from build123d import *

# Parameters (mm, degrees)
F2_R      = 51.5
F2_R_2    = 49
F5_DEPTH  = 10
F7_R      = 2.5
F8_DEPTH  = 5
F9_W      = 160.924614
F9_H      = 163.103462
F9_W_2    = 140
F9_H_2    = 140
F10_DEPTH = 10


with BuildPart() as f4:
    # F3 (on Front) → F4 (revolve)
    with BuildSketch(Plane.XZ):
        with BuildLine():
            ThreePointArc((63.105709, 14.230078), (67.468124, 7.701262), (69, 0))
            Line((69, 0), (72.5, 0))
            ThreePointArc((72.5, 0), (71.091539, 7.08081), (67.080583, 13.083631))
            Line((67.080583, 13.083631), (59.515611, 20.648602))
            ThreePointArc((59.515611, 20.648602), (53.58319, 29.527099), (51.5, 40))
            Line((51.5, 40), (45, 40))
            ThreePointArc((45, 40), (46.408461, 32.91919), (50.419417, 26.916369))
            Line((50.419417, 26.916369), (63.105709, 14.230078))
        make_face()
    revolve(axis=Axis((0, 0, 20), (0, 0, 1)))

    # F2 (on offset) → F5 (join)
    with BuildSketch(Plane.XY.offset(40)):
        Circle(F2_R)
        Circle(F2_R_2, mode=Mode.SUBTRACT)
    extrude(amount=F5_DEPTH)

    # F7 (on offset) → F8 (join)
    with BuildSketch(Plane.XY.offset(5)):
        with BuildLine():
            Line((-70, 65), (-70, 16.028423))
            ThreePointArc((-70, 16.028423), (-50.778491, 50.778491), (-16.028423, 70))
            Line((-16.028423, 70), (-65, 70))
            ThreePointArc((-65, 70), (-68.535534, 68.535534), (-70, 65))
        make_face()
        with Locations((-62.25, 62.25)):
            Circle(F7_R, mode=Mode.SUBTRACT)
        with BuildLine():
            ThreePointArc((-16.028423, -70), (-50.778491, -50.778491), (-70, -16.028423))
            Line((-70, -16.028423), (-70, -65))
            ThreePointArc((-70, -65), (-68.535534, -68.535534), (-65, -70))
            Line((-65, -70), (-16.028423, -70))
        make_face()
        with Locations((-62.25, -62.25)):
            Circle(F7_R, mode=Mode.SUBTRACT)
        with BuildLine():
            ThreePointArc((70, -16.028423), (50.778491, -50.778491), (16.028423, -70))
            Line((16.028423, -70), (65, -70))
            ThreePointArc((65, -70), (68.535534, -68.535534), (70, -65))
            Line((70, -65), (70, -16.028423))
        make_face()
        with Locations((62.25, -62.25)):
            Circle(F7_R, mode=Mode.SUBTRACT)
        with BuildLine():
            Line((65, 70), (16.028423, 70))
            ThreePointArc((16.028423, 70), (50.778491, 50.778491), (70, 16.028423))
            Line((70, 16.028423), (70, 65))
            ThreePointArc((70, 65), (68.535534, 68.535534), (65, 70))
        make_face()
        with Locations((62.25, 62.25)):
            Circle(F7_R, mode=Mode.SUBTRACT)
    extrude(amount=-F8_DEPTH)

    # F9 (on Top) → F10 (cut)
    with BuildSketch(Plane.XY):
        Rectangle(F9_W, F9_H)
        Rectangle(F9_W_2, F9_H_2, mode=Mode.SUBTRACT)
    extrude(amount=F10_DEPTH, mode=Mode.SUBTRACT)


solid = f4.part
Verification items for the finished model (mm, model axes). A direction names the side the tool comes from. Coordinates: 2 decimals unless noted, no trailing zeros. Order: outer loops, then holes, each group sorted by start corner. A loop starts at its lowest first (then second) coordinate and runs counter-clockwise, first axis right, second up.
Item 1: Material ranges on L1, parallel to Y at x = 62.25, z = 2.95; L2, parallel to Y at x = 62.25, z = 2.8; L3, parallel to Z at x = -59, y = 59, recorded low to high.
Filled in:
L1: y = -70 to -64.75, -59.75 to -29.26, 29.26 to 59.75, 64.75 to 70
L2: y = -70 to -64.75, -59.75 to -29.31, 29.31 to 59.75, 64.75 to 70
L3: z = 0 to 5
Item 2: Depth check by flat-ended pin: pin 1 (4 mm diameter, centred on x = 15.5, z = 9.5, fed in from +Y); pin 2 (2 mm diameter, centred on x = -35, y = -43.5, fed in from -Z); pin 3 (8 mm diameter, centred on x = 31, z = 11.5, fed in from +Y). Enter the tip coordinate at first touch or a pass-through.
Filled in:
pin 1: stops at y = 69.29
pin 2: stops at z = 20.5
pin 3: stops at y = 64.48
Item 3: Section check B-B, the plane z = 45. Enter the section's corners in (x, y).
Filled in:
outline: circle Ø103 at (0, 0); hole circle Ø98 at (0, 0)
Item 4: Release check for a two-part mould opening along Y. For faces 5 (the face through (23.632, -45.435, 26.123)), 6 (the face through (-47.52, -36.44, 20.28)), 7 (the face through (-47, -52, 0)) record: +Y half, -Y half, draft (parallel to the pull), parting line (faces both ways), or undercut.
Filled in:
face 5: undercut
face 6: parting line
face 7: draft
Item 5: Access from +Z, -Z, +X, -X, +Y, -Y to the whole of each face (thin tool, end or side, straight path). Record for faces 1 (the face through (64.635, -61.499, 2.535)), 2 (the face through (-57, -57, 5)), 3 (the face through (-55, 57, 5)), 4 (the face through (22, -40, 40)).
Filled in:
face 1: +Z, -Z
face 2: +Z, -X, -Y
face 3: +Z, -X, +Y
face 4: +Z
Item 6: Section check A-A, the plane y = 0. Enter the section's corners in (x, z), then the cut area to 3 significant figures.
Filled in:
outline: (-70, 0) - (-69, 0) arc R20.12 cw to (-63.11, 14.23) - (-50.42, 26.92) arc R18.5 ccw to (-45, 40) - (-49, 40) - (-49, 50) - (-51.5, 50) - (-51.5, 40) arc R27.37 cw to (-59.52, 20.65) - (-67.08, 13.08) arc R18.5 ccw to (-70, 9.29) - close; (45, 40) arc R18.5 ccw to (50.42, 26.92) - (63.11, 14.23) arc R20.12 cw to (69, 0) - (70, 0) - (70, 9.29) arc R18.5 ccw to (67.08, 13.08) - (59.52, 20.65) arc R27.37 cw to (51.5, 40) - (51.5, 50) - (49, 50) - (49, 40) - close
area: 346 mm2
Item 7: Section check C-C, the plane z = 29.5. Enter the section's corners in (x, y), then the cut area to 3 significant figures.
Filled in:
outline: circle Ø107.19 at (0, 0); hole circle Ø96.54 at (0, 0)
area: 1,700 mm2
